Study the drawing (mm; zero at the part's minimum x, y, z) and answer. A direction names the side the tool comes from. Round coordinates to 2 decimals unless told otherwise and drop trailing zeros. Write each loop counter-clockwise with the first axis right and the second up, starting at its lowest first coordinate (ties: lowest second). Pieces come first, ordered by that corner, then holes. Notation, with made-up numbers: (54, 56.25) - (63, 56.25) arc R15 cw to (63, 74.25) - close; hole circle Ø4 at (23.5, 43.25). An arc over 180 degrees is marked (long way). Return JSON: item names as keys, results as strings. Group by question number.
(1) Section B-B, the plane y = 52 is taken. Write down the section's boundary in (x, z), then the cut area to 3 significant figures.
(2) Section A-A, the plane x = 15 is taken. Write down the section's boundary in (y, z), then the cut area to 3 significant figures.
(3) Find the intervals of material crossed by line 1 along X through (y, z) = (15, 15.25); line 2 along X through (y, z) = (45, 14), in increasing order. Write a range as [from, to].
(4) Section C-C, the plane z = 15 is taken. Write down the section's boundary in (x, y), then the cut area to 3 significant figures.
(5) Section D-D, the plane z = 3.5 is taken. Write down the section's boundary in (x, y).
(6) Determine the mould class of the marked faces 1, 2, 3 and 4 for opening direction X: +X half, -X half, draft (parallel to the pull), parting line (faces both ways), or undercut.
(7) Which of the six approach directions +Z, -Z, +X, -X, +Y, -Y give full straight-line access (tool end or side, diameter ignored) to the marked faces 5, 6, 7, 8 and 9?
(8) Each of these flat-tipped pins is pushed along its axis until it touches: pin 1 (10.5 mm diameter, centred on x = 11, y = 50.5, fed in from -Z); pin 2 (5 mm diameter, centred on x = 22.5, z = 19, fed in from -Y); pin 3 (16 mm diameter, centred on x = 15, z = 15, fed in from -Y); pin 4 (10.5 mm diameter, centred on y = 52, z = 16, fed in from +X). Where does it stop, or does it pass through?
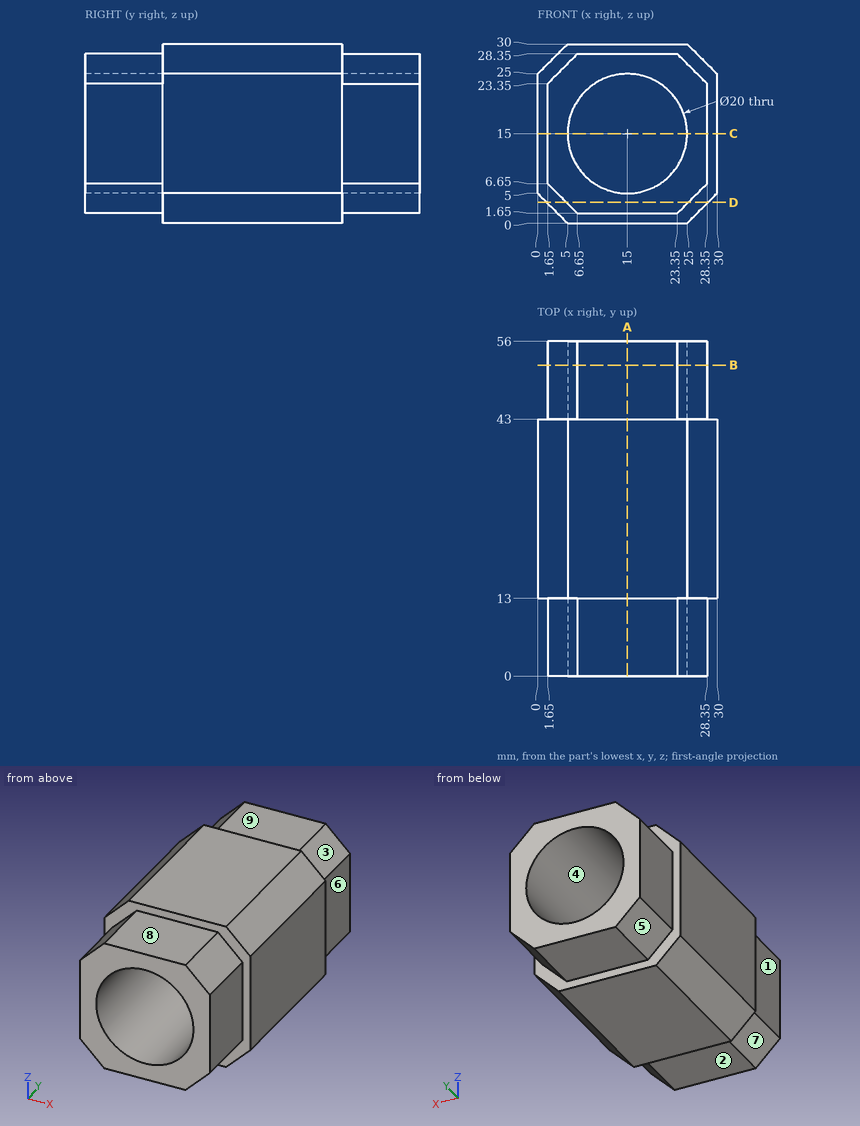
Working result:
{
 "1": {"outline": "(1.65, 6.65) - (6.65, 1.65) - (23.35, 1.65) - (28.35, 6.65) - (28.35, 23.35) - (23.35, 28.35) - (6.65, 28.35) - (1.65, 23.35) - close; hole circle Ø20 at (15, 15)", "area": "349 mm^2"},
 "2": {"outline": "(0, 1.65) - (13, 1.65) - (13, 0) - (43, 0) - (43, 1.65) - (56, 1.65) - (56, 5) - (0, 5) - close; (0, 25) - (56, 25) - (56, 28.35) - (43, 28.35) - (43, 30) - (13, 30) - (13, 28.35) - (0, 28.35) - close", "area": "474 mm^2"},
 "3": {"line 1": "x = [0, 5], [25, 30]", "line 2": "x = [1.65, 5.05], [24.95, 28.35]"},
 "4": {"outline": "(0, 13) - (1.65, 13) - (1.65, 0) - (5, 0) - (5, 56) - (1.65, 56) - (1.65, 43) - (0, 43) - close; (25, 0) - (28.35, 0) - (28.35, 13) - (30, 13) - (30, 43) - (28.35, 43) - (28.35, 56) - (25, 56) - close", "area": "474 mm^2"},
 "5": {"outline": "(1.5, 13) - (4.8, 13) - (4.8, 0) - (25.2, 0) - (25.2, 13) - (28.5, 13) - (28.5, 43) - (25.2, 43) - (25.2, 56) - (4.8, 56) - (4.8, 43) - (1.5, 43) - close"},
 "6": {"face 1": "-X half", "face 2": "draft", "face 3": "+X half", "face 4": "undercut"},
 "7": {"face 5": "-Z, -X, +Y", "face 6": "+Z, -Z, +X, +Y", "face 7": "-Z, -X, -Y", "face 8": "+Z, +X, -X, -Y", "face 9": "+Z, +X, -X, +Y"},
 "8": {"pin 1": "stops at z = 1.65", "pin 2": "stops at y = 0", "pin 3": "passes through", "pin 4": "stops at x = 28.35"}
}
